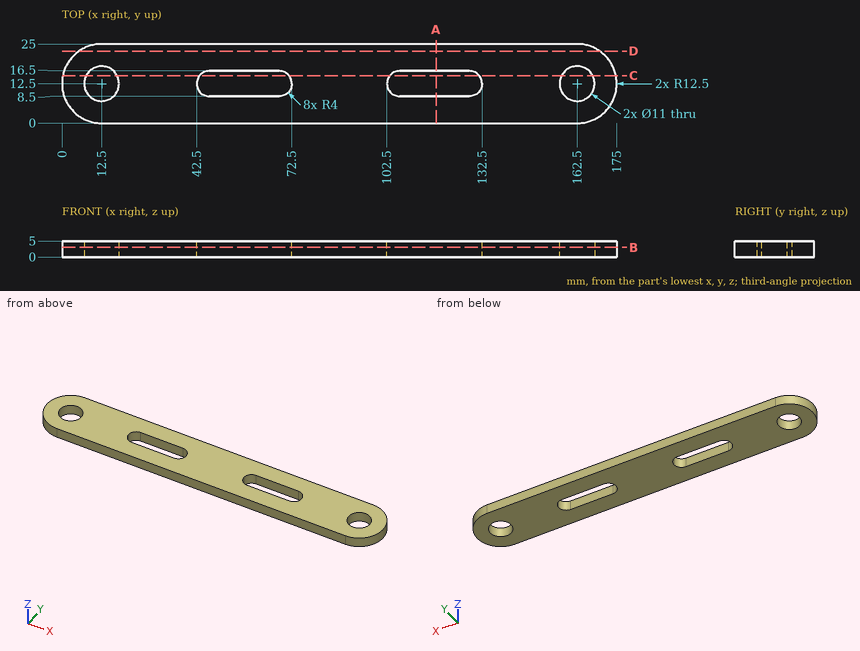
Job drawing, mm, ordinate dimensions from the low corner. One solid piece. Coordinates: 2 decimals unless noted, no trailing zeros. Order: outer loops, then holes, each group sorted by start corner. A loop starts at its lowest first (then second) coordinate and runs counter-clockwise, first axis right, second up. Notation, with made-up numbers: (36, 65) -> (41, 65) arc R22 ccw to (41, 71) -> close; hole circle Ø4 at (55, -20.75). An arc over 180 degrees is marked (long way). Put each result on its own line as item: value. Start each with the question number.
(1) Band-saw the part on C-C (y = 15). Give the cut face in (x, z), then the cut area to 3 significant figures.
(2) Band-saw the part on A-A (x = 118). Give the cut face in (y, z), then the cut area to 3 significant figures.
(3) Pin check, flat tips, straight feed: pin 1 Ø5 at (x, y) = (42.5, 15.5) entering from -Z; pin 2 Ø1 at (y, z) = (16.5, 2.5) entering from +X. Stop position of each tip, or through.
(4) Band-saw the part on D-D (y = 22.75). Give the cut face in (x, z).
(5) Band-saw the part on B-B (z = 3.1). Count the separate pieces of the cut face and the enclosed holes in it, then the cut area to 3 significant figures.
(6) Probe line 1 along Y through (x, z) = (162.5, 2.85); line 2 along Y through (x, z) = (54, 2.6); line 3 along X through (y, z) = (14.5, 2.65). List the from-to ranges inside material, lowest first. Write a range as [from, to].
Determined:
1. outline: (0.25, 0) -> (7.6, 0) -> (7.6, 5) -> (0.25, 5) -> close; (17.4, 0) -> (43.38, 0) -> (43.38, 5) -> (17.4, 5) -> close; (71.62, 0) -> (103.38, 0) -> (103.38, 5) -> (71.62, 5) -> close; (131.62, 0) -> (157.6, 0) -> (157.6, 5) -> (131.62, 5) -> close; (167.4, 0) -> (174.75, 0) -> (174.75, 5) -> (167.4, 5) -> close
1. area: 492 mm²
2. outline: (0, 0) -> (8.5, 0) -> (8.5, 5) -> (0, 5) -> close; (16.5, 0) -> (25, 0) -> (25, 5) -> (16.5, 5) -> close
2. area: 85.0 mm²
3. pin 1: stops at z = 0
3. pin 2: stops at x = 174.5
4. outline: (5.35, 0) -> (169.65, 0) -> (169.65, 5) -> (5.35, 5) -> close
5. separate pieces: 1
5. enclosed holes: 4
5. area: 3,600 mm²
6. line 1: y = [0, 7], [18, 25]
6. line 2: y = [0, 8.5], [16.5, 25]
6. line 3: x = [0.16, 7.38], [17.62, 43.04], [71.96, 103.04], [131.96, 157.38], [167.62, 174.84]
